```python
from build123d import *

# Parameters (mm, degrees)
SKETCH043_R  = 3.1
PAD035_DEPTH = 2.8
SKETCH044_R  = 3.1
PAD036_DEPTH = 2.8
FILLET001_R  = 1


with BuildPart() as part:
    # Sketch043 (on DatumPlane) → Pad035 (new body)
    with BuildSketch(Plane.YZ.offset(24.3)):
        with BuildLine():
            ThreePointArc((7.092358, 1.212106), (21.242166, -5.003536), (12.095894, 7.454272))
            Line((12.095894, 7.454272), (-16.105893, 30.059991))
            ThreePointArc((-16.105893, 30.059991), (-30.255701, 36.275633), (-21.109429, 23.817826))
            Line((7.092358, 1.212106), (-21.109429, 23.817826))
        make_face()
        with Locations((15, 0)):
            Circle(SKETCH043_R, mode=Mode.SUBTRACT)
        with Locations((-24.013535, 31.272097)):
            Circle(SKETCH043_R, mode=Mode.SUBTRACT)
    extrude(amount=PAD035_DEPTH)

    # Sketch044 (on Face8 of Pad035) → Pad036 (join)
    with BuildSketch(Plane.YZ.offset(27.1)):
        Polygon((-30.941816, 36.825603), (-32.675153, 29.317903), (-27.886115, 23.281752), (-20.180945, 23.262493), (-15.361794, 29.27463), (-17.05758, 36.790901), (-23.991342, 40.1514), align=None)
        with Locations((-24.013535, 31.272097)):
            Circle(SKETCH044_R, mode=Mode.SUBTRACT)
    extrude(amount=-PAD036_DEPTH)

    # Fillet001
    fillet001_edges = [part.edges().sort_by_distance(p)[0] for p in [
        (25.7, -15.413825, 29.50525),
        (25.7, -17.05758, 36.790901),
        (25.7, -23.991342, 40.1514),
        (25.7, -30.941816, 36.825603),
        (25.7, -32.675153, 29.317903),
        (25.7, -27.886115, 23.281752),
        (25.7, -20.417361, 23.263084),
    ]]
    fillet(fillet001_edges, radius=FILLET001_R)


solid = part.part
```
The listing builds one solid part. Answer for the finished solid, in the listing's coordinates (mm). Coordinates: 2 decimals unless noted, no trailing zeros. Write each loop counter-clockwise with the first axis right and the second up, starting at its lowest first coordinate (ties: lowest second). Pieces come first, ordered by that corner, then holes. Notation, with made-up numbers: (25, 15) - (66, 15) arc R35 cw to (66, 47) - close; hole circle Ø8 at (21.25, 46.25). An arc over 180 degrees is marked (long way). Return JSON: item names as keys, results as strings. Group by question number.
Q1. The part is cut by section D-D on z = 35. Write down the section's boundary in (x, y), and give its area (3 significant figures).
Q2. The part is cut by section C-C on x = 25.2. State how many separate pieces and enclosed holes the cut face has, and give its area (3 significant figures).
Q3. The part is cut by section A-A on z = 0. Write down the section's boundary in (x, y), and give its area (3 significant figures).
Q4. For a pull along Y with two mould halves and no side action, classify faces 1 (the cylindrical face through (25.68, -24.417, 34.346)), 2 (the flat face through (25.72, -18.985, 37.725)), 3 (the flat face through (24.3, -5, 14)) as +Y half, -Y half, draft (parallel to the pull), parting line (faces both ways), or undercut.
Q5. The part is cut by section B-B on y = 15. Write down the section's boundary in (x, z), and give its area (3 significant figures).
Q6. Find the intervals of material crossed by line 1 along Z through (x, y) = (26.05, 15); line 2 along Y through (x, z) = (26.45, 32); line 3 along Z through (x, y) = (25.25, -22.5), in increasing order. Write a range as [from, to].
Q7. Flat-ended cylindrical pins translate along their axes: pin 1 Ø1.5 at (x, y) = (25.5, -4) entering from -Z; pin 2 Ø5.5 at (y, z) = (15, 0) entering from +X. Find the tip coordinate at first contact, or state that the pin passes through.
Evaluation:
{
 "1": {"outline": "(24.3, -31.36) - (27.1, -31.36) - (27.1, -16.65) - (24.3, -16.65) - close", "area": "41.2 mm2"},
 "2": {"separate pieces": "1", "enclosed holes": "2", "area": "631 mm2"},
 "3": {"outline": "(24.3, 7) - (27.1, 7) - (27.1, 11.9) - (24.3, 11.9) - close; (24.3, 18.1) - (27.1, 18.1) - (27.1, 23) - (24.3, 23) - close", "area": "27.4 mm2"},
 "4": {"face 1": "undercut", "face 2": "+Y half", "face 3": "draft"},
 "5": {"outline": "(24.3, -8) - (27.1, -8) - (27.1, -3.1) - (24.3, -3.1) - close; (24.3, 3.1) - (27.1, 3.1) - (27.1, 8) - (24.3, 8) - close", "area": "27.4 mm2"},
 "6": {"line 1": "z = [-8, -3.1], [3.1, 8]", "line 2": "y = [-32.06, -27.03], [-21, -15.98]", "line 3": "z = [23.27, 28.57], [33.98, 39.43]"},
 "7": {"pin 1": "stops at z = 9.5", "pin 2": "passes through"}
}
